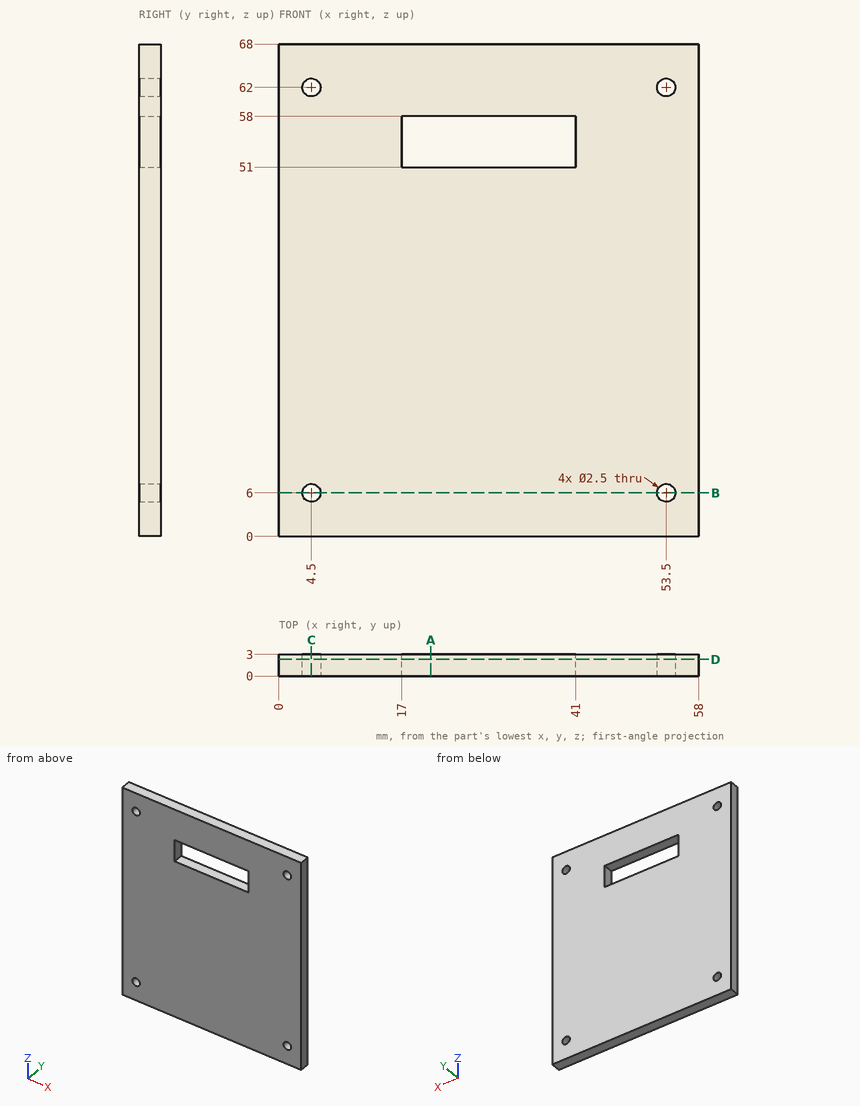
The figure shows three views and two pictorial views of one solid part (mm, origin at its lowest corner). Answer the questions. Coordinates: 2 decimals unless noted, no trailing zeros. Write each loop counter-clockwise with the first axis right and the second up, starting at its lowest first coordinate (ties: lowest second). Pieces come first, ordered by that corner, then holes. Notation, with made-up numbers: (23, 23) -> (66, 23) arc R8 ccw to (66, 32) -> close; hole circle Ø6 at (-11, 71). An arc over 180 degrees is marked (long way). Return JSON: item names as keys, results as strings.
(1) This flat-tipped pin is pushed along its axis until it touches: P1, Ø1.5, axis at y = 1.5, z = 46, coming from the -X side. Where does it stop, or does it pass through?
Answers below:
{"P1": "x = 0"}
(2) The part is cut by section D-D on y = 2.3. Give the vertices of the cut face in (x, z), then the cut area to 3 significant figures.
Answers below:
{"outline": "(0, 0) -> (58, 0) -> (58, 68) -> (0, 68) -> close; hole circle Ø2.5 at (4.5, 6); hole circle Ø2.5 at (4.5, 62); hole (17, 51) -> (41, 51) -> (41, 58) -> (17, 58) -> close; hole circle Ø2.5 at (53.5, 6); hole circle Ø2.5 at (53.5, 62)", "area": "3,760 mm^2"}
(3) Consider line 1 along X through (y, z) = (1.45, 6); line 2 along Z through (x, y) = (4.5, 2.35); line 3 along X through (y, z) = (1.1, 57). Determine where each line is inside the solid, lowest interval first. Write a range as from..to.
Answers below:
{"line 1": "0..3.25, 5.75..52.25, 54.75..58", "line 2": "0..4.75, 7.25..60.75, 63.25..68", "line 3": "0..17, 41..58"}
(4) The part is cut by section B-B on z = 6. Give the vertices of the cut face in (x, y), then the cut area to 3 significant figures.
Answers below:
{"outline": "(0, 0) -> (3.25, 0) -> (3.25, 3) -> (0, 3) -> close; (5.75, 0) -> (52.25, 0) -> (52.25, 3) -> (5.75, 3) -> close; (54.75, 0) -> (58, 0) -> (58, 3) -> (54.75, 3) -> close", "area": "159 mm^2"}
(5) The part is cut by section C-C on x = 4.5. Give the vertices of the cut face in (y, z), then the cut area to 3 significant figures.
Answers below:
{"outline": "(0, 0) -> (3, 0) -> (3, 4.75) -> (0, 4.75) -> close; (0, 7.25) -> (3, 7.25) -> (3, 60.75) -> (0, 60.75) -> close; (0, 63.25) -> (3, 63.25) -> (3, 68) -> (0, 68) -> close", "area": "189 mm^2"}
(6) The part is cut by section A-A on x = 21. Give the vertices of the cut face in (y, z), then the cut area to 3 significant figures.
Answers below:
{"outline": "(0, 0) -> (3, 0) -> (3, 51) -> (0, 51) -> close; (0, 58) -> (3, 58) -> (3, 68) -> (0, 68) -> close", "area": "183 mm^2"}
